Autodesk Inventor part; units mm, degrees
ref_plane "YZ Plane" through (0, 0, 0) normal (1, 0, 0) x (0, 1, 0)
ref_plane "XZ Plane" through (0, 0, 0) normal (0, 1, 0) x (-1, 0, 0)
ref_plane "XY Plane" through (0, 0, 0) normal (0, 0, 1) x (1, 0, 0)
sketch "Sketch1" plane through (0, 0, 0) normal (0, 1, 0) x (-1, 0, 0)
  line L0 (10, 6) -> (-70, 6)
  line L1 (-70, 6) -> (-70, -9)
  line L2 (-70, -9) -> (10, -9)
  line L3 (10, -9) -> (10, 6)
  line L4 (-17, -9) -> (-4, -22)
  line L5 (-4, -22) -> (10, -22)
  line L6 (10, -22) -> (10, -9)
  line L7 (-43, -9) -> (-56, -22)
  line L8 (-56, -22) -> (-70, -22)
  line L9 (-70, -22) -> (-70, -9)
  line L10 (-56, -22) -> (-4, -22)
  line L11 (-4, -22) -> (-4, -4)
  line L12 (-4, -4) -> (-56, -4)
  line L13 (-56, -4) -> (-56, -22)
  point P0 (0, 0)
  point P1 (-4, -22)
  dimension "d0" = 15
  dimension "d1" = 80
extrude "Extrusion1" add sketch "Sketch1" along normal blind 950 contours L3 L2 L11 L12 L13 L1 L0 | L6 L5 L11 L2 | L2 L13 L8 L9
properties part number "L_PlNKA800" material "Aluminum 6061"
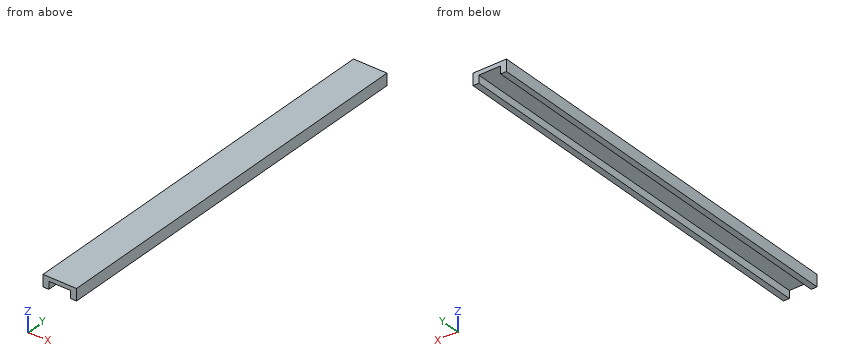
CAD build for the part. Positions are in the model's coordinates, mm. Give positions to 0.01 mm unless a question says otherwise; leave off trailing zeros. Order: outer loops, then holes, each group sorted by start corner. A loop starts at its lowest first (then second) coordinate and runs counter-clockwise, first axis right, second up. Notation, with made-up numbers: (-28, 56) - (-2, 56) arc R16 cw to (-2, 72) - close; hole circle Ø5 at (27.5, 20). An arc over 180 degrees is marked (long way). Answer in a Markdown table with one row per item.
1. Saw through at A-A, the plane z = -9.5. Give the cut face in (x, y).
Data:
| item | result |
|---|---|
| outline | (-10, 0) - (4, 0) - (4, 950) - (-10, 950) - close; (56, 0) - (70, 0) - (70, 950) - (56, 950) - close |
2. Probe probe 1 along X at (y, z) = (539, -17.5); probe 2 along Z at (x, y) = (33.5, 708). List the from-to ranges inside material, lowest first. Write a range as [from, to].
Data:
| item | result |
|---|---|
| probe 1 | x = [-10, 4], [56, 70] |
| probe 2 | z = [-4, 6] |
3. Saw through at C-C, the plane x = 19.5. Give the cut face in (y, z), plus the area to 3 significant figures.
Data:
| item | result |
|---|---|
| outline | (0, -4) - (950, -4) - (950, 6) - (0, 6) - close |
| area | 9,500 mm² |
4. Saw through at B-B, the plane y = 477.5. Give the cut face in (x, z), plus the area to 3 significant figures.
Data:
| item | result |
|---|---|
| outline | (-10, -22) - (4, -22) - (4, -4) - (56, -4) - (56, -22) - (70, -22) - (70, 6) - (-10, 6) - close |
| area | 1,300 mm² |
5. Flat gauge pin, fed straight in: pin 1 (3 mm diameter, centred on x = 6, y = 130, fed in from -Z). Where does the tip first touch, or does it go through?
Data:
| item | result |
|---|---|
| pin 1 | stops at z = -4 |
